Autodesk Inventor part; units mm, degrees
ref_plane "YZ Plane" through (0, 0, 0) normal (1, 0, 0) x (0, 1, 0)
ref_plane "XZ Plane" through (0, 0, 0) normal (0, 1, 0) x (-1, 0, 0)
ref_plane "XY Plane" through (0, 0, 0) normal (0, 0, 1) x (1, 0, 0)
sketch "Sketch1" plane through (0, 0, 0) normal (1, 0, 0) x (0, 1, 0)
  line L0 (0, 20.6375) -> (25.4, 20.6375)
  line L1 (0, 20.6375) -> (0, -54.5465)
  line L2 (0, -54.5465) -> (25.4, 20.6375)
  point P0 (0, 0)
  dimension "d0" = 25.4
  dimension "d1" = 75.184
extrude "Extrusion1" add sketch "Sketch1" along normal blind 114.3
sketch "Sketch2" plane through (0, 25.4, 20.6375) normal (0, 0.9474, -0.3201) x (1, 0, 0)
  line L0 (0, 79.3586) -> (0, 0)
  line L1 (0, 0) -> (114.3, 0)
  line L2 (114.3, 79.3586) -> (114.3, 0)
  line L3 (0, 79.3586) -> (114.3, 79.3586)
  line L4 (0, 0) -> (114.3, 0)
  line L5 (72.8666, 0) -> (69.7688, 0)
  line L6 (69.7688, 0) -> (69.7688, 61.9125)
  line L7 (69.7688, 61.9125) -> (72.8666, 61.9125)
  line L8 (72.8666, 61.9125) -> (72.8666, 0)
  line L9 (43.6373, 0) -> (40.4623, 0)
  line L10 (40.4623, 0) -> (40.4623, 61.9125)
  line L11 (40.4623, 61.9125) -> (43.6373, 61.9125)
  line L12 (43.6373, 61.9125) -> (43.6373, 0)
  point P0 (0, 27.6815)
  dimension "d4" = 3.175
extrude "Extrusion2" add sketch "Sketch2" along normal blind 25.4 contours L10 L11 L12 L1 | L1 L6 L7 L8
properties part number "WOODEN CORRECT SLIDER"
Verification items for the finished model (mm, model axes). A direction names the side the tool comes from. Round coordinates to 2 decimals unless told otherwise and drop trailing zeros. Order: outer loops, then holes, each group sorted by start corner. A loop starts at its lowest first (then second) coordinate and runs counter-clockwise, first axis right, second up. Notation, with made-up numbers: (29, -7.75) -> (72, -7.75) arc R25 ccw to (72, 10.25) -> close; hole circle Ø2 at (75, 46.5). An arc over 180 degrees is marked (long way). Put each result on its own line as item: value. Start each with the question number.
(1) Section check B-B (z = -24). Enter the section's corners in (x, y), then the cut area to 3 significant figures.
(2) Section check C-C (x = 60.5). Enter the section's corners in (y, z), then the cut area to 3 significant figures.
(3) Draft check along X on faces 6 (the face through (40.462, 27, -12)), 7 (the face through (43.637, 27, -13)), 8 (the face through (42.03, 37.26, 16.63)). Enter one of: +X half, -X half, draft (parallel to the pull), parting line (faces both ways), or undercut.
(4) Tool access check on faces 1 (the face through (71.296, 39.416, -17.231)), 2 (the face through (71.3, 37.26, 16.63)), 3 (the face through (72.867, 27, -13)), 4 (the face through (71.296, 17.446, -42.026)), 5 (the face through (69.769, 27, -12)). Record the directions out of +Z, -Z, +X, -X, +Y, -Y that give a thin tool (end or side, any length) a straight path to the whole face; none if there is none.
(5) Section check D-D (y = 15.5). Enter the section's corners in (x, z).
(6) Depth check by flat-ended pin: pin 1 Ø13 at (y, z) = (31.5, -20) entering from +X; pin 2 Ø22 at (y, z) = (31.5, -5.5) entering from -X; pin 3 Ø4 at (x, z) = (61, -31) entering from +Y. Enter the tip coordinate at first touch or a pass-through.
(7) Material ranges on line 1 along X through (y, z) = (17.5, -6); line 2 along Y through (x, z) = (90.5, -39); line 3 along Y through (x, z) = (55, -3), recorded low to high.
(8) Section check A-A (y = 42.5). Enter the section's corners in (x, z).
Completed:
1. outline: (0, 0) -> (114.3, 0) -> (114.3, 10.32) -> (72.87, 10.32) -> (72.87, 37.13) -> (69.77, 37.13) -> (69.77, 10.32) -> (43.64, 10.32) -> (43.64, 37.13) -> (40.46, 37.13) -> (40.46, 10.32) -> (0, 10.32) -> close
1. area: 1,350 mm2
2. outline: (0, -54.55) -> (25.4, 20.64) -> (0, 20.64) -> close
2. area: 955 mm2
3. face 6: -X half
3. face 7: undercut
3. face 8: draft
4. face 1: -Z, +X, -X, +Y
4. face 2: +Z, +X, -X, +Y
4. face 3: -Z, +X, +Y
4. face 4: -Z, +X, -X
4. face 5: -Z, +Y
5. outline: (0, -8.67) -> (40.46, -8.67) -> (40.46, -41.37) -> (43.64, -41.37) -> (43.64, -8.67) -> (69.77, -8.67) -> (69.77, -41.37) -> (72.87, -41.37) -> (72.87, -8.67) -> (114.3, -8.67) -> (114.3, 20.64) -> (0, 20.64) -> close
6. pin 1: stops at x = 72.87
6. pin 2: stops at x = 40.46
6. pin 3: stops at y = 8.63
7. line 1: x = 40.46 to 43.64, 69.77 to 72.87
7. line 2: y = 0 to 5.25
7. line 3: y = 0 to 17.41
8. outline: (40.46, -8.1) -> (43.64, -8.1) -> (43.64, 14.86) -> (40.46, 14.86) -> close; (69.77, -8.1) -> (72.87, -8.1) -> (72.87, 14.86) -> (69.77, 14.86) -> close
